CAD build for the part. Positions are in the model's coordinates, mm. A direction names the side the tool comes from. Round coordinates to 2 decimals unless told otherwise and drop trailing zeros. Loops run counter-clockwise (first coordinate to the right, second up) from the corner with the lowest first, then second, coordinate; pieces in that order, holes last. Notation, with made-up numbers: M 10,70.5 L 69,70.5 A21 cw 69,83.5 Z; hole C -7,28 d2. An arc over 180 degrees is marked long. Use one line per item in the form item = value.
from build123d import *

# Parameters (mm, degrees)
SKETCH_1_R               = 13.5
EXTRUDE_1_DEPTH          = 3
SKETCH_2_R               = 13.5
EXTRUDE_3_DEPTH          = 23
CUT_EXTRUDE_1_DEPTH      = 23
CUT_EXTRUDE_1_DEPTH_BACK = 23


with BuildPart() as part:
    # Sketch 1 → Extrude 1 (new body)
    with BuildSketch(Plane.XY):
        Circle(SKETCH_1_R)
        with BuildLine():
            Line((0, -2.832983292), (-4.900787729, -7.749547196))
            ThreePointArc((-4.900787729, -7.749547196), (-7.729211202, -7.754092383), (-7.733756389, -4.92566891))
            Line((-7.733756389, -4.92566891), (-2.828423473, -0.004545187))
            ThreePointArc((-2.828423473, -0.004545187), (-2.828427125, 0), (-2.828423473, 0.004545187))
            Line((-2.828423473, 0.004545187), (-7.733756389, 4.92566891))
            ThreePointArc((-7.733756389, 4.92566891), (-7.729211202, 7.754092383), (-4.900787729, 7.749547196))
            Line((-4.900787729, 7.749547196), (0, 2.832983292))
            Line((0, 2.832983292), (4.900787729, 7.749547196))
            ThreePointArc((4.900787729, 7.749547196), (7.729211202, 7.754092383), (7.733756389, 4.92566891))
            Line((7.733756389, 4.92566891), (2.828423473, 0.004545187))
            ThreePointArc((2.828423473, 0.004545187), (2.828427125, 0), (2.828423473, -0.004545187))
            Line((2.828423473, -0.004545187), (7.733756389, -4.92566891))
            ThreePointArc((7.733756389, -4.92566891), (7.729211202, -7.754092383), (4.900787729, -7.749547196))
            Line((4.900787729, -7.749547196), (0, -2.832983292))
        make_face(mode=Mode.SUBTRACT)
    extrude(amount=EXTRUDE_1_DEPTH)

    # Sketch 2 → Extrude 3 (add)
    with BuildSketch(Plane.XY.offset(3)):
        Circle(SKETCH_2_R)
        with BuildLine():
            ThreePointArc((-8.438592403, 4.216287709), (-8.435180773, 8.462334548), (-4.189144899, 8.452099668))
            Line((-4.189144899, 8.452099668), (-0.01808109, 4.25413827))
            Line((-0.01808109, 4.25413827), (4.198281258, 8.461255384))
            ThreePointArc((4.198281258, 8.461255384), (8.435180773, 8.462334548), (8.447718707, 4.225453447))
            Line((8.447718707, 4.225453447), (4.233699653, -0.025060575))
            Line((4.233699653, -0.025060575), (8.424997972, -4.243386968))
            ThreePointArc((8.424997972, -4.243386968), (8.414877485, -8.441965901), (4.216287709, -8.438592403))
            Line((4.216287709, -8.438592403), (0.036402841, -4.258707534))
            Line((0.036402841, -4.258707534), (-4.152452764, -8.483840182))
            ThreePointArc((-4.152452764, -8.483840182), (-8.469351133, -8.496614906), (-8.470450678, -4.179697776))
            Line((-8.470450678, -4.179697776), (-4.251903786, 0.029599093))
            Line((-4.251903786, 0.029599093), (-8.438592403, 4.216287709))
        make_face(mode=Mode.SUBTRACT)
    extrude(amount=EXTRUDE_3_DEPTH)

    # Sketch 4 → Cut-Extrude 1 (cut, two sides: drawn at the far end of the back side and taken through both)
    with BuildSketch(Plane(origin=(2.117926536, 2.10435635, 0), x_dir=(0, 0, 1), z_dir=(-0.7093757200092603, -0.7048305384000778, 0)).offset(-CUT_EXTRUDE_1_DEPTH_BACK)):
        with BuildLine():
            ThreePointArc((7.419819974, 3.030526502), (11.436613158, -6.154536667), (19.35, 0))
            ThreePointArc((19.35, 0), (19.154536667, 1.563386842), (18.580180026, 3.030526502))
            Line((18.580180026, 3.030526502), (7.419819974, 3.030526502))
        make_face()
        with BuildLine():
            Line((7.419819974, 3.030526502), (18.580180026, 3.030526502))
            ThreePointArc((18.580180026, 3.030526502), (13, 6.35), (7.419819974, 3.030526502))
        make_face()
    extrude(amount=CUT_EXTRUDE_1_DEPTH + CUT_EXTRUDE_1_DEPTH_BACK, mode=Mode.SUBTRACT)


solid = part.part
1. Cut at C-C on y = -3.75. State how many separate pieces and enclosed holes the cut face has, and give its area (3 significant figures).
Completed:
separate_pieces = 3
enclosed_holes = 0
area = 235 mm2
2. Probe line 1 along Y through (x, z) = (9, 4.25); line 2 along Y through (x, z) = (5.75, 24); line 3 along X through (y, z) = (2.5, 19.5). List the from-to ranges inside material, lowest first. Write a range as from..to.
Completed:
line_1 = -10.06..-7.61, -5.06..4.99, 7.68..10.06
line_2 = -12.21..-9.25, -1.55..1.5, 9.28..12.21
line_3 = -13.27..-6.72, 6.74..13.27
3. Drop flat-ended pins along their axis: P1, Ø2, axis at y = 6.5, z = 14.5, coming from the +X side; P2, Ø1, axis at x = -5.5, y = -2, coming from the +Z side; P3, Ø4, axis at y = -6.5, z = 14, coming from the +X side. Give the stop position or say it passes through.
Completed:
P1 = -1.13
P2 = 3
P3 = 12.73
4. Cut at D-D on z = 16.5. Write the cut outline in (x, y) (3 decimals).
Completed:
outline = M -12.543,-4.993 L -5.864,1.642 L -8.439,4.216 A3 cw -4.189,8.452 L -1.617,5.863 L 5.074,12.51 A13.5 ccw Z; M -5.074,-12.51 A13.5 ccw 12.543,4.993 L 5.852,-1.654 L 8.425,-4.243 A2.971 cw 4.216,-8.439 L 1.629,-5.851 Z
5. Cut at B-B on z = 4.75. Write the cut outline in (x, y) (3 decimals).
Completed:
outline = C 0,0 d27; hole M -8.47,-4.18 A3.048 ccw -4.152,-8.484 L 0.036,-4.259 L 4.216,-8.439 A2.971 ccw 8.425,-4.243 L 4.234,-0.025 L 8.448,4.225 A3 ccw 4.198,8.461 L -0.018,4.254 L -4.189,8.452 A3 ccw -8.439,4.216 L -4.252,0.03 Z
6. Pull direction X, two halves, no side cores. Call faces 3 (the face through (5.315, 2.5, 1.479)), 4 (the face through (6, 0, 26)), 5 (the face through (-6.391, -2.105, 5.176)), 6 (the face through (12.47, -5.17, 12.82)): +X half, -X half, draft (parallel to the pull), parting line (faces both ways), or undercut.
Completed:
face_3 = undercut
face_4 = draft
face_5 = undercut
face_6 = parting line
7. Tool access for faces 1 (the face through (-2.42, -5.26, 1.48)), 2 (the face through (6.37, 2.13, 22.25)): list every direction of +Z, -Z, +X, -X, +Y, -Y with a clear straight run to the whole face (end or side of a thin tool).
Completed:
face_1 = +Z, -Z
face_2 = +Z
8. Cut at A-A on z = 10. Write the cut outline in (x, y) (3 decimals), and give its area (3 significant figures).
Completed:
outline = M -12.66,-4.689 L -6.075,1.853 L -8.439,4.216 A3 cw -4.189,8.452 L -1.827,6.074 L 4.77,12.629 A13.5 ccw Z; M -4.77,-12.629 A13.5 ccw 12.66,4.689 L 6.063,-1.866 L 8.425,-4.243 A2.971 cw 4.216,-8.439 L 1.84,-6.062 Z
area = 211 mm2
